Source: CAD feature listing. Evaluate the final solid. Frame: model axes, mm. Round coordinates to 2 decimals unless told otherwise and drop trailing zeros. Order: outer loops, then holes, each group sorted by start corner. A loop starts at its lowest first (then second) coordinate and runs counter-clockwise, first axis right, second up. Notation, with made-up numbers: (85.25, 87) - (104.25, 87) arc R19 cw to (104.25, 117) - close; hole circle Ø11 at (25, 13). An arc over 180 degrees is marked (long way). Put each result on its own line as item: value. Start each with the question number.
1) Contact query for flat-ended pins moving along their axis: P1, Ø1.6, axis at y = 0.5, z = 2, coming from the +X side; P2, Ø0.6, axis at y = 1, z = 3, coming from the +X side; P3, Ø1.6, axis at x = -25.5, y = 0.5, coming from the +Z side. Output: stop coordinate, or through.
2) Section C-C on z = 37. Output: boundary loops of the cut face in (x, y), then the cut area to 3 significant figures.
3) Section B-B on x = -6. Output: boundary loops of the cut face in (y, z).
4) Line query: probe 1 along Z at (x, y) = (-61, 1); probe 2 along X at (y, z) = (1, 10); probe 3 along X at (y, z) = (-4.25, 24). Output: solid intervals per line, ascending. Write a range as [from, to].
5) Section A-A on y = -5. Output: boundary loops of the cut face in (x, z).
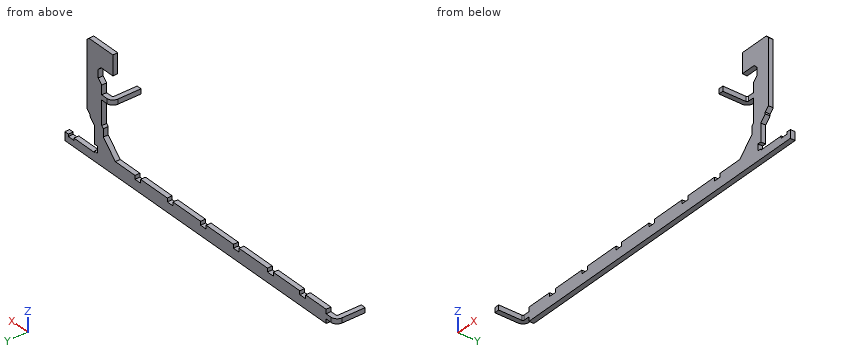
```python
from build123d import *

# Parameters (mm, degrees)
BOSS_EXTRUDE1_DEPTH     = 2
EDGE_FLANGE1_DEPTH      = 2
EDGE_FLANGE1_BEND_DEPTH = 2
MOVE_FACE1_BY           = 5
CUT_EXTRUDE1_DEPTH      = 10


# Sheet-metal steps are written as plain solids
with BuildPart() as part:
    # Sketch1 → Boss-Extrude1 (new body)
    with BuildSketch(Plane(origin=(0, 0, 0), x_dir=(1, 0, 0), z_dir=(0, 1, 0))):
        Polygon((48.786990623, -23.171897133), (48.786990623, -13.328634875), (47.986992223, -12.528636475), (47.986992223, -9.428635055), (41.786991923, -3.228634755), (-54.913007717, -3.228634755), (-66.471417942, -3.228634755), (-66.471417942, -1.378635375), (-68.471417942, -1.378635375), (-68.471417942, 0.621364625), (-66.471417942, 0.621364625), (-66.471417942, 2.471364005), (-54.913007717, 2.471364005), (65.786992183, 2.471364005), (65.786992183, -1.128636415), (52.786992783, -1.128636415), (52.786992783, -11.528635935), (54.986990923, -13.728634075), (54.986993463, -14.428635215), (56.686992603, -16.128634355), (56.686992603, -42.528634895), (53.786993323, -45.428634175), (43.086991863, -45.428634175), (43.086991863, -34.028634115), (49.286992163, -34.028634115), (50.586992103, -32.728634175), (50.586992103, -30.828635435), (48.786990623, -29.028636495), (48.786990623, -25.171897133), (46.786990623, -25.171897133), (46.786990623, -23.171897133), align=None)
    extrude(amount=BOSS_EXTRUDE1_DEPTH)

    # Edge-Flange1 section (across the edge) → Edge-Flange1 (add)
    with BuildSketch(Plane(origin=(-69.471417942, 0, 1.378635375), x_dir=(1, 0, 0), z_dir=(0, 0, -1))):
        with BuildLine():
            Line((-2, 0.5), (-2, 10))
            Line((-2, 10), (0, 10))
            Line((0, 10), (0, 0.5))
            ThreePointArc((0, 0.5), (0.146446609, 0.146446609), (0.5, 0))
            Line((0.5, 0), (1, 0))
            Line((1, 0), (1, -2))
            Line((1, -2), (0.5, -2))
            ThreePointArc((0.5, -2), (-1.267766953, -1.267766953), (-2, 0.5))
        make_face()
    extrude(amount=EDGE_FLANGE1_DEPTH)

    # Edge-Flange1 section 2 (across the edge) → Edge-Flange1 bend (add)
    with BuildSketch(Plane(origin=(45.786990623, 0, 25.171897133), x_dir=(1, 0, 0), z_dir=(0, 0, -1))):
        with BuildLine():
            Line((-2, 0.5), (-2, 10))
            Line((-2, 10), (0, 10))
            Line((0, 10), (0, 0.5))
            ThreePointArc((0, 0.5), (0.146446609, 0.146446609), (0.5, 0))
            Line((0.5, 0), (1, 0))
            Line((1, 0), (1, -2))
            Line((1, -2), (0.5, -2))
            ThreePointArc((0.5, -2), (-1.267766953, -1.267766953), (-2, 0.5))
        make_face()
    extrude(amount=EDGE_FLANGE1_BEND_DEPTH)

    # Move Face1: a face moved outward by 5.0
    extrude(part.faces().sort_by_distance((65.786992183, 1, -0.671363795))[0], amount=MOVE_FACE1_BY, dir=(1, 0, 0))

    # Sketch12 → Cut-Extrude1 (cut)
    with BuildSketch(Plane(origin=(0, 2, 0), x_dir=(1, 0, 0), z_dir=(0, 1, 0))):
        Polygon((-52.913012042, -1.628639718), (-55.913012042, -1.628639718), (-55.913012042, -3.128639258), (-67.564249917, -3.128639258), (-67.671952829, -4.327104706), (41.886988858, -5.326407077), (48.086989158, -13.828640718), (48.007739716, -22.517187069), (46.286990623, -23.171897133), (48.886987558, -23.171897133), (48.886987558, -13.328639178), (48.086989158, -12.528640778), (48.086989158, -9.328639558), (41.886988858, -3.128639258), (31.786988738, -3.128639258), (31.786988738, -1.628639718), (28.886989458, -1.628639718), (28.886989458, -3.128639258), (15.186988918, -3.128639258), (15.186988918, -1.628639718), (12.286989638, -1.628639718), (12.286989638, -3.128639258), (-1.913012442, -3.128639258), (-1.913012442, -1.628639718), (-4.813011722, -1.628639718), (-4.813011722, -3.128639258), (-18.813011662, -3.128639258), (-18.813011662, -1.628639718), (-21.713010942, -1.628639718), (-21.713010942, -3.128639258), (-36.313012222, -3.128639258), (-36.313012222, -1.628639718), (-39.313011302, -1.628639718), (-39.313011302, -3.128639258), (-52.913012042, -3.128639258), align=None)
        Polygon((48.886987558, -25.171897133), (46.286990623, -25.171897133), (41.570815933, -34.028638418), (41.570815933, -47.167587605), (56.254650903, -46.954291818), (57.278434149, -42.02008581), (58.126913923, -16.761088184), (54.30540669, -8.580570975), (54.30540669, -2.3223377), (71.613193797, -2.589733287), (71.946410025, 3.760976012), (44.354427072, 3.760976012), (-68.474759816, 3.760976012), (-68.386329283, 2.371359902), (67.886988718, 2.371359902), (67.886988718, -1.028638378), (66.086988718, -1.028638378), (66.086988718, -0.128640178), (63.186989438, -0.128640178), (63.186989438, -1.028638378), (52.686987578, -1.028638378), (52.686987578, -1.528639918), (51.186988038, -1.528639918), (51.186988038, -4.228639598), (52.686987578, -4.228639598), (52.686987578, -11.528640238), (54.986988058, -13.828640718), (54.986988058, -14.528639318), (56.586989938, -16.128641198), (56.586989938, -42.428636858), (55.486987058, -43.528639738), (43.186988798, -43.528639738), (43.186988798, -35.428640698), (49.286986758, -35.428640698), (50.686989038, -34.028638418), (50.686989038, -30.728637398), (48.886987558, -28.928638458), align=None)
    extrude(amount=-CUT_EXTRUDE1_DEPTH, mode=Mode.SUBTRACT)


solid = part.part
```
Answer sheet:
1. P1: x = 52.69
1. P2: x = 51.19
1. P3: z = 3.13
2. outline: (43.19, 0) - (56.59, 0) - (56.59, 2) - (43.19, 2) - close
2. area: 26.8 mm^2
3. outline: (0, -2.37) - (2, -2.37) - (2, 3.13) - (0, 3.13) - close
4. probe 1: [-2.37, 3.13]
4. probe 2: [48.09, 52.69]
4. probe 3: [43.79, 45.79]
5. outline: (-71.47, -0.62) - (-69.47, -0.62) - (-69.47, 1.38) - (-71.47, 1.38) - close; (43.79, 23.17) - (45.79, 23.17) - (45.79, 25.17) - (43.79, 25.17) - close
